```python
from build123d import *

# Parameters (mm, degrees)
F1_DEPTH      = 42
F2_R          = 1.5
F3_DEPTH      = 25.001
F3_DEPTH_BACK = 90
F6_DEPTH      = 25


# Not quite as in the source:
# - an extrude ends at something that could not be found from the text; its depth is read off the source's solid


with BuildPart() as f1:
    # F0 (on Top) → F1 (new body)
    with BuildSketch(Plane.XY):
        with BuildLine():
            Line((-12.622932768, 0), (-7.5127989985, 0))
            Line((-7.5127989985, 0), (-7.5127989985, 8))
            ThreePointArc((-7.5127989985, 8), (-17.257361645, 9.7445626465), (-19.0019242916, 0))
            Line((-19.0019242916, 0), (-13.8917905221, 0))
            ThreePointArc((-13.8917905221, 0), (-15.8872915916, 7.0799299466), (-9.207361645, 4))
            ThreePointArc((-9.207361645, 4), (-10.1774316984, 1.3700700534), (-12.622932768, 0))
        make_face()
        with BuildLine():
            ThreePointArc((-6.257361645, 4), (-6.5785916039, 1.9038056538), (-7.5127989985, 0))
            Line((-7.5127989985, 0), (-2.5127989985, 0))
            Line((-2.5127989985, 0), (-2.5127989985, 8))
            Line((-2.5127989985, 8), (-7.5127989985, 8))
            ThreePointArc((-7.5127989985, 8), (-6.5785916039, 6.0961943462), (-6.257361645, 4))
        make_face()
        with BuildLine():
            Line((-7.5127989985, 8), (-7.5127989985, 0))
            ThreePointArc((-7.5127989985, 0), (-6.5785916039, 1.9038056538), (-6.257361645, 4))
            ThreePointArc((-6.257361645, 4), (-6.5785916039, 6.0961943462), (-7.5127989985, 8))
        make_face()
        with BuildLine():
            Line((-2.5127989985, 8), (-2.5127989985, 0))
            Line((-2.5127989985, 0), (5.4872010015, 0))
            Line((5.4872010015, 0), (5.4872010015, 20))
            Line((5.4872010015, 20), (17.7872010015, 20))
            Line((17.7872010015, 20), (17.7872010015, 0))
            Line((17.7872010015, 0), (22.7872010015, 0))
            Line((22.7872010015, 0), (22.7872010015, 20))
            ThreePointArc((22.7872010015, 20), (21.3227349074, 23.5355339059), (17.7872010015, 25))
            Line((17.7872010015, 25), (-2.5127989985, 25))
            Line((-2.5127989985, 25), (-2.5127989985, 8))
        make_face()
    extrude(amount=F1_DEPTH)

    # F2 (on Front) → F3 (cut, two sides)
    with BuildSketch(Plane.XZ) as f3_sk:
        with BuildLine():
            Line((-20.1659295708, 21), (-20.1659295708, 38.6531305723))
            ThreePointArc((-20.1659295708, 38.6531305723), (-37.8190601431, 21), (-20.1659295708, 3.3468694277))
            Line((-20.1659295708, 3.3468694277), (-20.1659295708, 21))
        make_face()
        with BuildLine():
            ThreePointArc((-20.1659295708, 3.3468694277), (-7.683281234, 8.5173516632), (-2.5127989985, 21))
            Line((-2.5127989985, 21), (-20.1659295708, 21))
            Line((-20.1659295708, 21), (-20.1659295708, 3.3468694277))
        make_face()
        with Locations((0, 38.2)):
            Circle(F2_R)
        with Locations((0, 5.3)):
            Circle(F2_R)
        with BuildLine():
            Line((-20.1659295708, 21), (-2.5127989985, 21))
            ThreePointArc((-2.5127989985, 21), (-7.683281234, 33.4826483368), (-20.1659295708, 38.6531305723))
            Line((-20.1659295708, 38.6531305723), (-20.1659295708, 21))
        make_face()
    extrude(amount=-F3_DEPTH, mode=Mode.SUBTRACT)
    extrude(f3_sk.sketch, amount=F3_DEPTH_BACK, mode=Mode.SUBTRACT)

    # F5 (on offset) → F6 (cut)
    with BuildSketch(Plane.YZ.offset(10)):
        with BuildLine():
            ThreePointArc((4.1718953289, 5.5), (5.2325555007, 5.9393398282), (5.6718953289, 7))
            ThreePointArc((5.6718953289, 7), (3.1112351571, 8.0606601718), (4.1718953289, 5.5))
        make_face()
        with BuildLine():
            ThreePointArc((4.1718953289, 36.5), (3.1112351571, 33.9393398282), (5.6718953289, 35))
            ThreePointArc((5.6718953289, 35), (5.2325555007, 36.0606601718), (4.1718953289, 36.5))
        make_face()
    extrude(amount=F6_DEPTH, mode=Mode.SUBTRACT)


solid = f1.part
```
Work out the finished part from the listing and answer in its coordinate system (mm). A direction names the side the tool comes from. Round coordinates to 2 decimals unless told otherwise and drop trailing zeros. Write each loop counter-clockwise with the first axis right and the second up, starting at its lowest first coordinate (ties: lowest second). Pieces come first, ordered by that corner, then holes. Notation, with made-up numbers: (-34.75, 16.25) -> (-28.75, 16.25) arc R37 cw to (-28.75, 54.25) -> close; hole circle Ø8 at (64, 81.5). An arc over 180 degrees is marked (long way). Write each question's results on one line, items separated by ' | '.
Q1. Which of the six approach directions +Z, -Z, +X, -X, +Y, -Y give full straight-line access (tool end or side, diameter ignored) to faces 1 (the cylindrical face through (-14.902, 10.804, 39.525)), 2 (the flat face through (-4, 8, 36)), 3 (the flat face through (5.487, 10, 21))?
Data:
face 1: +Z, -Z | face 2: +Z, -Z, +Y | face 3: +Z, -Z, -Y
Q2. Section D-D, the plane x = -15.5 is taken. Write down the section's boundary in (y, z).
Data:
outline: (0, 0) -> (0.63, 0) -> (0.63, 3.97) -> (0, 3.97) -> close; (0, 38.03) -> (0.63, 38.03) -> (0.63, 42) -> (0, 42) -> close; (7.37, 0) -> (10.63, 0) -> (10.63, 3.97) -> (7.37, 3.97) -> close; (7.37, 38.03) -> (10.63, 38.03) -> (10.63, 42) -> (7.37, 42) -> close
Q3. Determine the mould class of faces 4 (the cylindrical face through (-14.902, 10.804, 2.353)), 5 (the flat face through (22.787, 10, 21)), 6 (the flat face through (1, 13, 0)) for opening direction X: released by +X, released by -X, zero draft, split by the parting line, or undercut.
Data:
face 4: undercut | face 5: released by +X | face 6: zero draft
Q4. Straight lines are drawn through the part: line 1 along Z through (x, y) = (0, 22); line 2 along X through (y, z) = (9.5, 15.5); line 3 along Y through (x, z) = (12.5, 6). For each, find the intervals that lie inside material, in ascending order. Write a range as [from, to].
Data:
line 1: [0, 3.8], [6.8, 36.7], [39.7, 42] | line 2: [-2.51, 5.49], [17.79, 22.79] | line 3: [20, 25]
Q5. Section C-C, the plane y = 7 is taken. Write down the section's boundary in (x, z).
Data:
outline: (-19.58, 0) -> (-15.98, 0) -> (-15.98, 3.85) arc R17.65 cw to (-19.58, 3.36) -> close; (-19.58, 38.64) arc R17.65 cw to (-15.98, 38.15) -> (-15.98, 42) -> (-19.58, 42) -> close; (-10.54, 0) -> (5.49, 0) -> (5.49, 42) -> (-10.54, 42) -> (-10.54, 35.8) arc R17.65 cw to (-10.54, 6.2) -> close; (17.79, 0) -> (22.79, 0) -> (22.79, 42) -> (17.79, 42) -> close; hole circle Ø3 at (0, 5.3); hole circle Ø3 at (0, 38.2)
Q6. Section B-B, the plane x = 0 is taken. Write down the section's boundary in (y, z).
Data:
outline: (0, 0) -> (25, 0) -> (25, 3.8) -> (0, 3.8) -> close; (0, 6.8) -> (25, 6.8) -> (25, 36.7) -> (0, 36.7) -> close; (0, 39.7) -> (25, 39.7) -> (25, 42) -> (0, 42) -> close
Q7. Section A-A, the plane y = 18 is taken. Write down the section's boundary in (x, z), then the cut area to 3 significant figures.
Data:
outline: (-2.51, 0) -> (5.49, 0) -> (5.49, 42) -> (-2.51, 42) -> close; (17.79, 0) -> (22.79, 0) -> (22.79, 42) -> (17.79, 42) -> close; hole circle Ø3 at (0, 5.3); hole circle Ø3 at (0, 38.2) | area: 532 mm^2
Q8. Flat-ended cylindrical pins translate along their axes: P1, Ø6, axis at y = 6.5, z = 26, coming from the -X side; P2, Ø12, axis at x = 10, y = 10, coming from the +Z side; P3, Ø1.5, axis at y = 15.5, z = 36.5, coming from the -X side; P4, Ø10, axis at x = 11.5, z = 26.5, coming from the -Y side. Find the tip coordinate at first contact, or state that the pin passes through.
Data:
P1: x = -4.43 | P2: z = 42 | P3: x = -2.51 | P4: y = 20
